from build123d import *

# Parameters (mm, degrees)
EXTRUDE_THIN1_DEPTH = 512
SKETCH3_R           = 4.5
CUT_EXTRUDE1_DEPTH  = 10
LPATTERN1_COUNT     = 4
LPATTERN1_PITCH     = 40
SKETCH4_W           = 116
SKETCH4_H           = 6
CUT_EXTRUDE2_DEPTH  = 6


with BuildPart() as part:
    # Sketch1 → Extrude-Thin1 (new body)
    with BuildSketch(Plane.XY):
        with BuildLine():
            Line((44, -6), (456, -6))
            ThreePointArc((456, -6), (491.355339059, 8.644660941), (506, 44))
            Line((506, 44), (506, 457))
            ThreePointArc((506, 457), (491.355339059, 492.355339059), (456, 507))
            Line((456, 507), (44, 507))
            ThreePointArc((44, 507), (8.644660941, 492.355339059), (-6, 457))
            Line((-6, 457), (-6, 44))
            ThreePointArc((-6, 44), (8.644660941, 8.644660941), (44, -6))
        make_face()
        with BuildLine():
            Line((44, 0), (456, 0))
            ThreePointArc((456, 0), (487.112698372, 12.887301628), (500, 44))
            Line((500, 44), (500, 457))
            ThreePointArc((500, 457), (487.112698372, 488.112698372), (456, 501))
            Line((456, 501), (44, 501))
            ThreePointArc((44, 501), (12.887301628, 488.112698372), (0, 457))
            Line((0, 457), (0, 44))
            ThreePointArc((0, 44), (12.887301628, 12.887301628), (44, 0))
        make_face(mode=Mode.SUBTRACT)
    extrude(amount=-EXTRUDE_THIN1_DEPTH)

    # Sketch3 → Cut-Extrude1 (cut)
    with BuildSketch(Plane(origin=(506, 0, 0), x_dir=(0, 0, -1), z_dir=(1, 0, 0))):
        with Locations((482, 407)):
            Circle(SKETCH3_R)
    cut_extrude1 = extrude(amount=-CUT_EXTRUDE1_DEPTH, mode=Mode.SUBTRACT)

    # LPattern1: Cut-Extrude1 ×4
    with Locations(*[(0, 0, i * LPATTERN1_PITCH) for i in range(1, LPATTERN1_COUNT)]):
        add(cut_extrude1, mode=Mode.SUBTRACT)

    # Sketch4 → Cut-Extrude2 (cut)
    with BuildSketch(Plane(origin=(0, 0, -512), x_dir=(-1, 0, 0), z_dir=(0, 0, -1))):
        with Locations((-250, 504)):
            Rectangle(SKETCH4_W, SKETCH4_H)
    extrude(amount=-CUT_EXTRUDE2_DEPTH, mode=Mode.SUBTRACT)


solid = part.part
The model under review builds one solid part; all positions refer to its coordinate system, in mm. A direction names the side the tool comes from. Round coordinates to 2 decimals unless told otherwise and drop trailing zeros. Loops run counter-clockwise (first coordinate to the right, second up) from the corner with the lowest first, then second, coordinate; pieces in that order, holes last. Notation, with made-up numbers: M 50.5,74.25 L 61.5,74.25 A35 ccw 61.5,107.25 Z; hole C 53.5,-23 d8. An arc over 180 degrees is marked long. Answer as CSV lines item,"result". Start each with the question number.
Item 1: Mouldability with a two-part tool opening along X and no side actions: class faces 3 (the face through (487.45, 487.77, -252.42)), 4 (the face through (491.742, 491.964, -252.416)), 5 (the face through (253, 507, -252)), 6 (the face through (9.036, 492.742, -252.416)) as released by +X, released by -X, zero draft, split by the parting line, or undercut.
Item 2: Consider section B-B (y = 237). Write out the cut boundary in (x, z), then the cut area to 3 significant figures.
Item 3: Insertion check: P1, Ø3, axis at y = 503.5, z = -509.5, coming from the +X side; P2, Ø3, axis at x = 259.5, y = 505, coming from the -Z side; P3, Ø7, axis at y = 407, z = -442, coming from the +X side. Each pin has a flat end and moves straight along its axis. Give the tip position at first contact, or say it passes through.
Item 4: Consider section A-A (x = 357.5). Write out the cut boundary in (y, z).
Item 5: For faces 1 (the face through (0, 253, -252)), 2 (the face through (-6, 253, -252)), list the 3-axis set-ups (+Z, -Z, +X, -X, +Y, -Y) from which the entire face can be reached by the end or side of a thin tool; tool diameter is ignored.
Item 6: Consider section C-C (z = -262.5). Write out the cut boundary in (x, y).
Item 7: Wall thickness on line 1 (Z direction, x = 502, y = 407); line 2 (Y direction, x = 66.5, z = -181); line 3 (X direction, y = 423, z = -206.5): over which ranges is each line inside the solid? List them lowest first. Write a range as [from, to].
Answer:
1,face 3,"undercut"
1,face 4,"released by +X"
1,face 5,"zero draft"
1,face 6,"released by -X"
2,outline,"M -6,-512 L 0,-512 L 0,0 L -6,0 Z; M 500,-512 L 506,-512 L 506,0 L 500,0 Z"
2,area,"6,140 mm^2"
3,P1,"stops at x = 477.79"
3,P2,"stops at z = -506"
3,P3,"stops at x = 0"
4,outline,"M -6,-512 L 0,-512 L 0,0 L -6,0 Z; M 501,-512 L 507,-512 L 507,0 L 501,0 Z"
5,face 1,"+Z, -Z"
5,face 2,"+Z, -Z, -X, +Y, -Y"
6,outline,"M -6,44 A50 ccw 44,-6 L 456,-6 A50 ccw 506,44 L 506,457 A50 ccw 456,507 L 44,507 A50 ccw -6,457 Z; hole M 0,44 A44 ccw 44,0 L 456,0 A44 ccw 500,44 L 500,457 A44 ccw 456,501 L 44,501 A44 ccw 0,457 Z"
7,line 1,"z = [-512, -486.5], [-477.5, -446.5], [-437.5, -406.5], [-397.5, -366.5], [-357.5, 0]"
7,line 2,"y = [-6, 0], [501, 507]"
7,line 3,"x = [-6, 0], [500, 506]"
